Here's how the part is built. I have some questions about the finished solid (model axes, mm). A direction names the side the tool comes from. Give positions to 0.01 mm unless a question says otherwise; leave off trailing zeros. Loops run counter-clockwise (first coordinate to the right, second up) from the corner with the lowest first, then second, coordinate; pieces in that order, holes last. Notation, with made-up numbers: (-8, -10.75) - (10, -10.75) arc R19 cw to (10, 26.25) - close; hole circle Ø4 at (31.5, 27). An arc over 180 degrees is marked (long way). Return JSON: item names as keys, results as strings. Group by question number.
(1) If we section it at A-A (y = 1.25): Please give me the cut outline in (x, z).
(2) If we section it at D-D (x = 85.5): Please give me the cut outline in (y, z).
(3) If we mould it in two halves opening along Z, with no side actions, what happens to faces 3 (the flat face through (15.4, 2, -4)), 4 (the cylindrical face through (13.59, 2.32, -10.49)), 5 (the flat face through (0.95, 2, 1))? For each: released by +Z, released by -Z, zero draft, split by the parting line, or undercut.
(4) For P1, Ø2, axis at y = 2.5, z = -22, coming from the -X side; P2, Ø2.5, axis at y = 3.5, z = -3, coming from the -X side; P3, Ø1.5, axis at x = -75, y = 1, coming from the -Z side; P4, Ø12, axis at x = -20.5, z = -1, coming from the -Y side, each with a flat end and sliding along its axis, tell me the tip position at first contact or that it passes through.
(5) If we section it at B-B (z = -10): Please give me the cut outline in (x, y), then the cut area to 3 significant figures.
(6) I need wall thicknesses on probe 1 along Z at (x, y) = (75, 2.65); probe 2 along X at (y, z) = (2.45, -7); probe 3 along X at (y, z) = (2.1, -9). Which ranges of each line are inside material? Lowest first, please. Write a range as [from, to].
(7) If we section it at C-C (x = 45): Please give me the cut outline in (y, z).
(8) On a 3-axis mill with a long thin cutter (end or side, diameter ignored), from which of +Z, -Z, +X, -X, +Y, -Y can I reach the whole of each face in a straight line? I mean faces 1 (the cylindrical face through (-8.09, 2.32, -10.59)), 2 (the flat face through (116.14, 2.25, -4.29)). Say none if no direction works.
```python
from build123d import *

# Parameters (mm, degrees)
BOSS_EXTRUDE1_DEPTH = 4.572
FILLET3_R           = 6.35
FILLET2_R           = 6.35


with BuildPart() as part:
    # Sketch1 → Boss-Extrude1 (new body)
    with BuildSketch(Plane(origin=(0, 0, 0), x_dir=(1, 0, 0), z_dir=(0, 1, 0))):
        Polygon((15.4, 12.401654114), (15.4, 0.971654114), (78.9, 0.971654114), (108.87813576, 30.949789874), (133.871024484, 30.949789874), (133.871024484, 22.022678598), (97.95, -13.898345886), (15.4, -13.898345886), (-10, -13.898345886), (-92.55, -13.898345886), (-128.471024484, 22.022678598), (-128.471024484, 30.949789874), (-103.47813576, 30.949789874), (-73.5, 0.971654114), (-10, 0.971654114), (-10, 12.401654114), align=None)
        with BuildLine():
            Line((0.95, -7.548345886), (0.95, 6.051654114))
            ThreePointArc((0.95, 6.051654114), (2.7, 7.801654114), (4.45, 6.051654114))
            Line((4.45, 6.051654114), (4.45, -7.548345886))
            ThreePointArc((4.45, -7.548345886), (2.7, -9.298345886), (0.95, -7.548345886))
        make_face(mode=Mode.SUBTRACT)
    extrude(amount=BOSS_EXTRUDE1_DEPTH)

    # Fillet3
    # the kernel refuses this fillet: 6.35 mm, written as the material it takes off along each edge
    with BuildSketch(Plane(origin=(133.871024484, -15.875, -30.949789874), x_dir=(0, 0, 1), z_dir=(0, 1, 0)), Plane(origin=(-128.471024484, -15.875, -30.949789874), x_dir=(1, 0, 0), z_dir=(0, 1, 0))) as fillet3_piece_1:
        with BuildLine():
            CenterArc((FILLET3_R, -FILLET3_R), FILLET3_R, 90, 90)
            Line((0, -FILLET3_R), (0, 0))
            Line((0, 0), (FILLET3_R, 0))
        make_face()
    extrude(amount=36.322, mode=Mode.SUBTRACT)
    with BuildSketch(Plane(origin=(-128.471024484, -6.575640303, -22.022678598), x_dir=(0, 0, -1), z_dir=(0, 1, 0)), Plane(origin=(133.871024484, -6.575640303, -22.022678598), x_dir=(-0.7071067811865476, 0, 0.7071067811865476), z_dir=(0, 1, 0)), Plane(origin=(97.95, -6.575640303, 13.898345886), x_dir=(-1, 0, 0), z_dir=(0, 1, 0)), Plane(origin=(-92.55, -6.575640303, 13.898345886), x_dir=(-0.7071067811865476, 0, -0.7071067811865476), z_dir=(0, 1, 0))) as fillet3_piece_2:
        with BuildLine():
            CenterArc((FILLET3_R * 0.414213562373, -FILLET3_R), FILLET3_R, 90, 45)
            Line((-FILLET3_R * 0.292893218813, -FILLET3_R * 0.292893218813), (0, 0))
            Line((0, 0), (FILLET3_R * 0.414213562373, 0))
        make_face()
    extrude(amount=17.723280605, mode=Mode.SUBTRACT)

    # Fillet2
    fillet2_edges = [part.edges().sort_by_distance(p)[0] for p in [
        (-10, 2.286, -12.401654114),
        (15.4, 2.286, -12.401654114),
    ]]
    fillet(fillet2_edges, radius=FILLET2_R)


solid = part.part
```
Values:
{
 "1": {"outline": "(-128.47, -24.63) arc R6.35 ccw to (-122.12, -30.95) - (-103.48, -30.95) - (-73.5, -0.97) - (-10, -0.97) - (-10, -6.05) arc R6.35 ccw to (-3.65, -12.4) - (9.05, -12.4) arc R6.35 ccw to (15.4, -6.05) - (15.4, -0.97) - (78.9, -0.97) - (108.88, -30.95) - (127.52, -30.95) arc R6.35 ccw to (133.87, -24.63) arc R6.35 ccw to (132.01, -20.16) - (99.81, 12.04) arc R6.35 ccw to (95.32, 13.9) - (-89.92, 13.9) arc R6.35 ccw to (-94.41, 12.04) - (-126.61, -20.16) arc R6.35 ccw to start; hole (0.95, -6.05) arc R1.75 ccw to (4.45, -6.05) - (4.45, 7.55) arc R1.75 ccw to (0.95, 7.55) - close"},
 "2": {"outline": "(0, -7.57) - (4.57, -7.57) - (4.57, 13.9) - (0, 13.9) - close"},
 "3": {"face 3": "zero draft", "face 4": "released by -Z", "face 5": "undercut"},
 "4": {"P1": "x = -128.25", "P2": "x = -110.7", "P3": "z = -3.22", "P4": "y = 0"},
 "5": {"outline": "(-116.45, 0) - (-82.53, 0) - (-82.53, 4.57) - (-116.45, 4.57) - close; (-8.62, 0) - (14.02, 0) - (14.02, 4.57) - (-8.62, 4.57) - close; (87.93, 0) - (121.85, 0) - (121.85, 4.57) - (87.93, 4.57) - close", "area": "414 mm2"},
 "6": {"probe 1": "[-0.97, 13.9]", "probe 2": "[-113.45, -79.53], [-9.93, 1.23], [4.17, 15.33], [84.93, 118.85]", "probe 3": "[-115.45, -81.53], [-9.27, 14.67], [86.93, 120.85]"},
 "7": {"outline": "(0, -0.97) - (4.57, -0.97) - (4.57, 13.9) - (0, 13.9) - close"},
 "8": {"face 1": "-Z, +Y, -Y", "face 2": "+Z, +X, +Y, -Y"}
}
